The drawing under review shows one solid part. Ordinate dimensions are in mm from its lowest x, y, z. Give positions to 0.01 mm unless a question says otherwise; leave off trailing zeros. Loops run counter-clockwise (first coordinate to the right, second up) from the corner with the lowest first, then second, coordinate; pieces in that order, holes last. Notation, with made-up numbers: M 25.5,-16 L 76.5,-16 A12 cw 76.5,-4 Z; hole C 41,-19.5 d1. An arc over 180 degrees is marked long. Put each result on its own line as item: value. Start each with the question number.
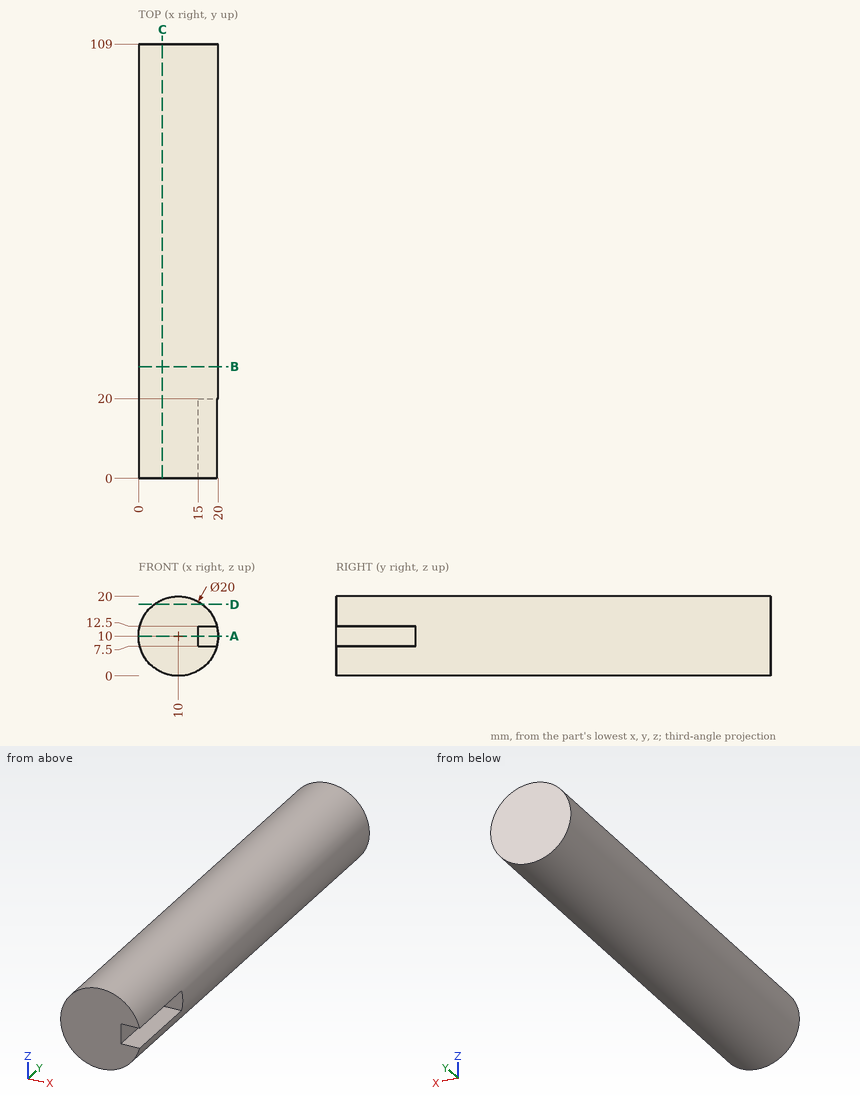
Item 1: To check wall thickness, follow L1, parallel to Y at x = 17, z = 10.75; L2, parallel to Z at x = 6.5, y = 82; L3, parallel to X at y = 48, z = 17.75. State the ranges of each line that lie inside material, in increasing order. Write a range as [from, to].
Item 2: Clearance check with flat-ended pins moving along their axes: pin 1 Ø1 at (x, y) = (6.5, 56.5) entering from -Z; pin 2 Ø8 at (y, z) = (52.5, 8) entering from +X; pin 3 Ø5 at (x, y) = (16.5, 94.5) entering from +Z; pin 4 Ø1.5 at (y, z) = (59, 6) entering from -X. State where each tip first meets the part, or that it passes through.
Item 3: Consider section D-D, the plane z = 18. Write out the cut boundary in (x, y).
Item 4: Consider section B-B, the plane y = 28. Write out the cut boundary in (x, z), plus the area to 3 significant figures.
Item 5: Consider section A-A, the plane z = 10. Write out the cut boundary in (x, y), plus the area to 3 significant figures.
Item 6: Consider section C-C, the plane x = 6. Write out the cut boundary in (y, z), plus the area to 3 significant figures.
Report:
1. L1: [20, 109]
1. L2: [0.63, 19.37]
1. L3: [3.68, 16.32]
2. pin 1: z = 0.46
2. pin 2: x = 20
2. pin 3: z = 19.17
2. pin 4: x = 0.54
3. outline: M 4,0 L 16,0 L 16,109 L 4,109 Z
4. outline: C 10,10 d20
4. area: 314 mm²
5. outline: M 0,0 L 15,0 L 15,20 L 20,20 L 20,109 L 0,109 Z
5. area: 2,080 mm²
6. outline: M 0,0.83 L 109,0.83 L 109,19.17 L 0,19.17 Z
6. area: 2,000 mm²
